Verification items for the finished model (mm, model axes). Give positions to 0.01 mm unless a question says otherwise; leave off trailing zeros. Loops run counter-clockwise (first coordinate to the right, second up) from the corner with the lowest first, then second, coordinate; pieces in that order, holes last. Notation, with made-up numbers: (63.25, -5) - (86.25, -5) arc R22 cw to (86.25, 18) - close; hole circle Ø4 at (12.5, 73). An arc over 180 degrees is marked (long way). Use one line per item in the form item = value.
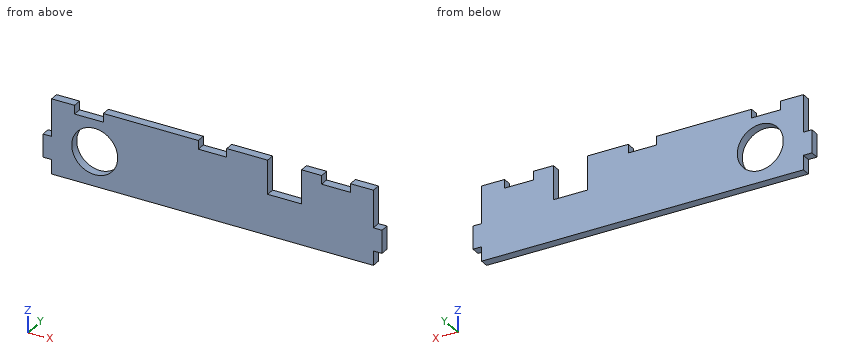
```python
from build123d import *

# Parameters (mm, degrees)
SKETCH1_R           = 8
BOSS_EXTRUDE1_DEPTH = 3


with BuildPart() as part:
    # Sketch1 → Boss-Extrude1 (new body)
    with BuildSketch(Plane(origin=(0, 0, 0), x_dir=(1, 0, 0), z_dir=(0, 1, 0))):
        Polygon((1213.408125786, -2432.393668664), (1216.408125786, -2432.393668664), (1216.408125786, -2424.393668664), (1213.408125786, -2424.393668664), (1213.408125786, -2419.393668664), (1101.408125786, -2419.393668664), (1101.408125786, -2424.393668664), (1098.408125786, -2424.393668664), (1098.408125786, -2432.393668664), (1101.408125786, -2432.393668664), (1101.408125786, -2445.393668664), (1109.408125786, -2445.393668664), (1109.408125786, -2442.393668664), (1119.408125786, -2442.393668664), (1119.408125786, -2445.393668664), (1152.458125786, -2445.393668664), (1152.458125786, -2442.393668664), (1162.358125786, -2442.393668664), (1162.358125786, -2445.393668664), (1176.608125786, -2445.393668664), (1176.608125786, -2433.593668664), (1188.408125786, -2433.593668664), (1188.408125786, -2445.393668664), (1195.408125786, -2445.393668664), (1195.408125786, -2442.393668664), (1205.408125786, -2442.393668664), (1205.408125786, -2445.393668664), (1213.408125786, -2445.393668664), align=None)
        with Locations((1116.408125786, -2431.393668664)):
            Circle(SKETCH1_R, mode=Mode.SUBTRACT)
    extrude(amount=BOSS_EXTRUDE1_DEPTH)


solid = part.part
```
1. Section check C-C, the plane x = 1161. Record the cut outline in (y, z), then the cut area to 3 significant figures.
Result set:
outline = (0, 2419.39) - (3, 2419.39) - (3, 2442.39) - (0, 2442.39) - close
area = 69.0 mm²
2. Section check B-B, the plane z = 2436. Record the cut outline in (x, y), then the cut area to 3 significant figures.
Result set:
outline = (1101.41, 0) - (1109.87, 0) - (1109.87, 3) - (1101.41, 3) - close; (1122.95, 0) - (1176.61, 0) - (1176.61, 3) - (1122.95, 3) - close; (1188.41, 0) - (1213.41, 0) - (1213.41, 3) - (1188.41, 3) - close
area = 261 mm²
3. Scan lines: probe 1 along X at (y, z) = (0.9, 2444); probe 2 along X at (y, z) = (0.5, 2441.75); probe 3 along X at (y, z) = (1.3, 2435.5). Record each from-to range of solid material in increasing order.
Result set:
probe_1 = 1101.41 to 1109.41, 1119.41 to 1152.46, 1162.36 to 1176.61, 1188.41 to 1195.41, 1205.41 to 1213.41
probe_2 = 1101.41 to 1176.61, 1188.41 to 1213.41
probe_3 = 1101.41 to 1109.54, 1123.27 to 1176.61, 1188.41 to 1213.41
4. Depth check by flat-ended pin: pin 1 Ø0.9 at (y, z) = (1, 2443) entering from +X; pin 2 Ø0.9 at (x, y) = (1180, 1.5) entering from +Z; pin 3 Ø13 at (x, z) = (1116.41, 2431.39) entering from +Y; pin 4 Ø0.9 at (y, z) = (1, 2440) entering from -X. Enter the tip coordinate at first touch or a pass-through.
Result set:
pin_1 = 1213.41
pin_2 = 2433.59
pin_3 = through
pin_4 = 1101.41
5. Section check D-D, the plane z = 2422.25. Record the cut outline in (x, y).
Result set:
outline = (1101.41, 0) - (1213.41, 0) - (1213.41, 3) - (1101.41, 3) - close
